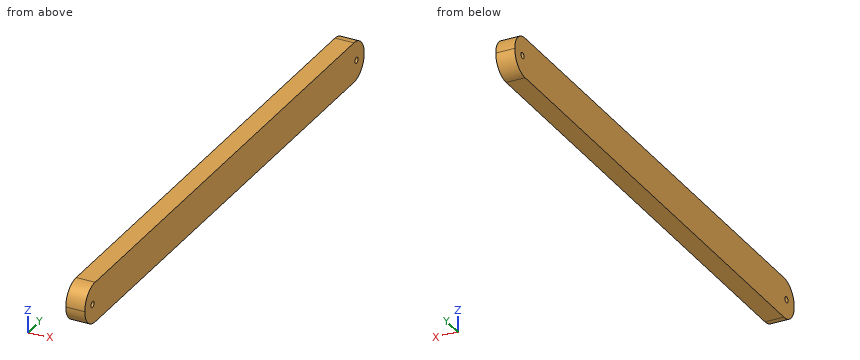
```python
from build123d import *

# Parameters (mm, degrees)
F0_W     = 540
F0_H     = 40
F0_R     = 3
F1_DEPTH = 19
F2_R     = 19.99999


# Not quite as in the source:
# - a fillet or chamfer is up to 0.001 mm smaller than in the source, because OpenCascade refuses the exact size


with BuildPart() as f1:
    # F0 (on Right) → F1 (new body)
    with BuildSketch(Plane.YZ):
        with Locations((-255, 0)):
            Rectangle(F0_W, F0_H)
        with Locations((-510, 0)):
            Circle(F0_R, mode=Mode.SUBTRACT)
        Circle(F0_R, mode=Mode.SUBTRACT)
    extrude(amount=F1_DEPTH)

    # F2 (radius 20 in the source; OpenCascade refuses exactly that, so slightly less here)
    f2_edges = [f1.edges().sort_by_distance(p)[0] for p in [
        (9.5, 15, 20),
        (9.5, 15, -20),
        (9.5, -525, 20),
        (9.5, -525, -20),
    ]]
    fillet(f2_edges, radius=F2_R)


solid = f1.part
```
Can you work these out from the model? Positions are in its coordinate system, mm. Coordinates: 2 decimals unless noted, no trailing zeros. Write item = value, one per line. Start each with the question number.
Q1. If we section it at A-A, the plane x = 15.75: State how many separate pieces and enclosed holes the cut face has, then the cut area to 3 significant figures.
Q2. I'm going to push a flat-ended pin straight in: pin 1 (8 mm diameter, centred on x = 13.5, z = 10, fed in from -Y). Where does the tip first touch, or does it pass through?
Q3. If I drill on L1, parallel to Z at x = 12.75, y = -510; L2, parallel to Y at x = 17.25, z = -1; L3, parallel to Y at x = 4.5, z = -12.5, over which ranges is the centre line in solid material (lowest first)? Write a range as [from, to].
Check sheet entries:
q1.separate_pieces = 1
q1.enclosed_holes = 2
q1.area = 21,200 mm²
q2.pin_1 = -524.08
q3.L1 = [-19.36, -3], [3, 19.36]
q3.L2 = [-524.97, -512.83], [-507.17, -2.83], [2.83, 14.97]
q3.L3 = [-520.61, 10.61]
